```python
from build123d import *

# Parameters (mm, degrees)
F2_R     = 6.7823339415
F3_DEPTH = 8.07
F4_R     = 5.9
F5_DEPTH = 1
F5_TAPER = 80


# Not quite as in the source:
# - an extrude ends at something that could not be found from the text; its depth is read off the source's solid


with BuildPart() as f1:
    # F0 (on Front) → F1 (revolve)
    with BuildSketch(Plane.XZ):
        with BuildLine():
            Line((12.1487583965, 8.07), (5.9, 8.07))
            Line((5.9, 8.07), (5.9, 1.82))
            Line((5.9, 1.82), (2.7476675302, 0))
            Line((2.7476675302, 0), (8.43, 0))
            Line((8.43, 0), (12.5, 4.07))
            ThreePointArc((12.5, 4.07), (12.4588304791, 6.0818062209), (12.1487583965, 8.07))
        make_face()
    revolve(axis=Axis((0, 0, -0.4323393759), (0, 0, 1)))

    # F2 (on face) → F3 (join, through all)
    with BuildSketch(Plane.XY.offset(8.07)):
        Circle(F2_R)
        Polygon((-5.9755752861, 0), (-2.9877876431, 5.175), (2.9877876431, 5.175), (5.9755752861, 0), (2.9877876431, -5.175), (-2.9877876431, -5.175), align=None, mode=Mode.SUBTRACT)
    extrude(amount=-F3_DEPTH)

    # F4 (on face) → F5 (cut)
    with BuildSketch(Plane.XY.offset(8.07)):
        Circle(F4_R)
    extrude(amount=-F5_DEPTH, taper=F5_TAPER, mode=Mode.SUBTRACT)


solid = f1.part
```
The listing builds one solid part. Answer for the finished solid, in the listing's coordinates (mm). A direction names the side the tool comes from. Give positions to 0.01 mm unless a question says otherwise; leave off trailing zeros. Answer in a Markdown table with one row per item. Add a question column.
Q1. Find the intervals of material crossed by line 1 along Y through (x, z) = (5.75, 6.5); line 2 along X through (y, z) = (1.5, 1.75); line 3 along X through (y, z) = (0.5, 4), in increasing order. Write a range as [from, to].
Q2. Which of the six approach directions +Z, -Z, +X, -X, +Y, -Y give full straight-line access (tool end or side, diameter ignored) to faces 4 (the flat face through (4.462, 2.622, 4.782)), 5 (the flat face through (-6, -3, 8.07))?
Q3. Given P1, Ø4.5, axis at x = 1, z = 4.5, coming from the -Y side; P2, Ø3, axis at y = 2.5, z = 1, coming from the +X side; P3, Ø4, axis at y = 1.5, z = 2.5, coming from the -X side, each flat-ended and moving along its own axis, determine where each tip first touches the part or whether it passes through.
Q4. For a pull along X with two mould halves and no side action, classify faces 1 (the flat face through (0, -4, 0)), 2 (the conical face through (-4.7, 2.76, 7.99)), 3 (the conical face through (-1.883, -8.478, 0.255)) as released by +X, released by -X, zero draft, split by the parting line, or undercut.
Determined:
| question | item | result |
|---|---|---|
| 1 | line 1 | y = [-11, -0.39], [0.39, 11] |
| 1 | line 2 | x = [-10.07, -5.11], [5.11, 10.07] |
| 1 | line 3 | x = [-12.42, -5.69], [5.69, 12.42] |
| 2 | face 4 | +Z |
| 2 | face 5 | +Z, +X, -X, +Y, -Y |
| 3 | P1 | stops at y = -12.52 |
| 3 | P2 | stops at x = 10.68 |
| 3 | P3 | stops at x = -12.5 |
| 4 | face 1 | zero draft |
| 4 | face 2 | undercut |
| 4 | face 3 | split by the parting line |
